Autodesk Inventor part; units mm, degrees
ref_plane "YZ Plane" through (0, 0, 0) normal (1, 0, 0) x (0, 1, 0)
ref_plane "XZ Plane" through (0, 0, 0) normal (0, 1, 0) x (-1, 0, 0)
ref_plane "XY Plane" through (0, 0, 0) normal (0, 0, 1) x (1, 0, 0)
sketch "Sketch1" plane through (0, 0, 0) normal (0, 0, 1) x (1, 0, 0)
  line L0 (-27.3, -5) -> (21, -5)
  line L1 (21, 0) -> (-27.3, 0)
  line L2 (-27.3, 0) -> (-27.3, -5)
  line L3 (17.4, 46.3236) -> (17.4, 0)
  line L4 (17.4, 0) -> (21, 0)
  line L5 (21, 41.8826) -> (21, 41.2832)
  line L6 (17.4, 46.3236) -> (21, 46.3236)
  line L7 (21, 46.3236) -> (21, 0)
  line L8 (21, 0) -> (17.4, 0)
  line L9 (17.4, 0) -> (17.4, 46.3236)
  line L10 (21, 0) -> (21, -5)
  point P0 (0, 0)
  point P1 (-27.3, 0)
  point P2 (17.4, 38.1655)
extrude "Extrusion1" add sketch "Sketch1" against normal blind 15
sketch "Sketch2" plane through (0, 0, 0) normal (0, 0, 1) x (1, 0, 0)
  line L0 (17.4, 0) -> (-27.3, 0)
  line L1 (-27.3, 0) -> (-27.3, -5)
  line L2 (21, -5) -> (21, 46.3236)
  line L3 (21, 46.3236) -> (17.4, 46.3236)
  line L4 (17.4, 46.3236) -> (17.4, 0)
  line L5 (-27.3, -5) -> (21, -5)
  point P0 (0, 0)
extrude "Extrusion2" add sketch "Sketch2" along normal blind 2
sketch "Sketch3" plane through (17.4, 0, -15) normal (-1, 0, 0) x (0, 0, 1)
  line L0 (10.8285, 34.887) -> (11.0682, 35.4658)
  line L1 (11.15, 36.087) -> (11.0682, 35.4658)
  line L2 (11.0682, 36.7082) -> (11.15, 36.087)
  line L3 (10.8285, 37.287) -> (11.0682, 36.7082)
  line L4 (10.4471, 37.7841) -> (10.8285, 37.287)
  line L5 (9.95, 38.1655) -> (10.4471, 37.7841)
  line L6 (9.3712, 38.4052) -> (9.95, 38.1655)
  line L7 (9.3712, 38.4052) -> (8.75, 38.487)
  line L8 (8.1288, 38.4052) -> (8.75, 38.487)
  line L9 (8.1288, 38.4052) -> (7.55, 38.1655)
  line L10 (7.55, 38.1655) -> (7.0529, 37.7841)
  line L11 (7.0529, 37.7841) -> (6.6715, 37.287)
  line L12 (6.6715, 37.287) -> (6.4318, 36.7082)
  line L13 (6.4318, 36.7082) -> (6.35, 36.087)
  line L14 (6.35, 36.087) -> (6.4318, 35.4658)
  line L15 (6.4318, 35.4658) -> (6.6715, 34.887)
  line L16 (6.6715, 34.887) -> (7.0529, 34.3899)
  line L17 (7.0529, 34.3899) -> (7.55, 34.0085)
  line L18 (8.1288, 33.7688) -> (7.55, 34.0085)
  line L19 (8.1288, 33.7688) -> (8.75, 33.687)
  line L20 (8.75, 33.687) -> (9.3712, 33.7688)
  line L21 (9.3712, 33.7688) -> (9.95, 34.0085)
  line L22 (9.95, 34.0085) -> (10.4471, 34.3899)
  line L23 (10.8285, 34.887) -> (10.4471, 34.3899)
  line L24 (8.75, 35.087) -> (9.0088, 35.1211)
  line L25 (8.4912, 35.1211) -> (8.75, 35.087)
  line L26 (8.25, 35.221) -> (8.4912, 35.1211)
  line L27 (8.0429, 35.3799) -> (8.25, 35.221)
  line L28 (7.884, 35.587) -> (8.0429, 35.3799)
  line L29 (7.7841, 35.8282) -> (7.884, 35.587)
  line L30 (7.75, 36.087) -> (7.7841, 35.8282)
  line L31 (7.7841, 36.3458) -> (7.75, 36.087)
  line L32 (7.884, 36.587) -> (7.7841, 36.3458)
  line L33 (8.0429, 36.7941) -> (7.884, 36.587)
  line L34 (8.25, 36.953) -> (8.0429, 36.7941)
  line L35 (8.4912, 37.0529) -> (8.25, 36.953)
  line L36 (8.75, 37.087) -> (8.4912, 37.0529)
  line L37 (8.75, 37.087) -> (9.0088, 37.0529)
  line L38 (9.0088, 37.0529) -> (9.25, 36.953)
  line L39 (9.25, 36.953) -> (9.4571, 36.7941)
  line L40 (9.4571, 36.7941) -> (9.616, 36.587)
  line L41 (9.616, 36.587) -> (9.7159, 36.3458)
  line L42 (9.7159, 36.3458) -> (9.75, 36.087)
  line L43 (9.75, 36.087) -> (9.7159, 35.8282)
  line L44 (9.7159, 35.8282) -> (9.616, 35.587)
  line L45 (9.616, 35.587) -> (9.4571, 35.3799)
  line L46 (9.4571, 35.3799) -> (9.25, 35.221)
  line L47 (9.25, 35.221) -> (9.0088, 35.1211)
  circle A0 centre (8.75, 36.087) radius 2.5
  arc A1 (12.25, 29.4537) -> (5.25, 29.4537) centre (8.75, 36.087) ccw
  line L48 (8.75, 36.087) -> (8.75, 28.587)
  line L49 (0, 0) -> (17, 0)
  line L50 (0, -5) -> (0, 0)
  line L51 (0, -5) -> (17, -5)
  line L52 (17, 0) -> (17, -5)
  line L53 (8.75, 28.587) -> (8.75, 0)
  line L54 (0, 0) -> (17, 0)
  line L55 (5.25, 14.2935) -> (5.25, 28.587)
  line L56 (12.25, 28.587) -> (12.25, 14.2935)
  line L57 (12.25, 0) -> (5.25, 0)
  line L58 (5.25, 0) -> (12.25, 28.587) construction
  line L59 (5.25, 28.587) -> (12.25, 0) construction
  line L60 (12.25, 28.587) -> (12.25, 29.4537)
  line L61 (5.25, 28.587) -> (5.25, 29.4537)
  line L62 (0, 46.3236) -> (17, 46.3236)
  line L63 (17, 46.3236) -> (0, 46.3236)
  line L64 (0, 46.3236) -> (0, 0)
  line L65 (0, 0) -> (17, 0)
  line L66 (17, 0) -> (17, 46.3236)
  line L67 (5.25, 14.2935) -> (0, 0)
  line L68 (12.25, 14.2935) -> (17, 0)
  point P0 (15, 0)
  point P1 (8.75, 14.2935)
  dimension "d6" = 5
  dimension "d7" = 15
  dimension "d8" = 7
extrude "Extrusion3" cut sketch "Sketch3" against normal up to surface (3.6 mm away) contours L25 L26 L27 L28 L29 L30 L31 L32 L33 L34 L35 L36 L37 L38 L39 L40 L41 L42 L43 L44 L45 L46 L47 L24 | L23 L22 L21 L20 L19 L18 L17 L16 L15 L14 L13 L12 L11 L10 L9 L8 L7 L6 L5 L4 L3 L2 L1 L0 | L64 L62 L66 L68 L56 L60 A1 L61 L55 L67
sketch "Sketch5" plane through (-27.3, -5, -15) normal (0, -1, 0) x (1, 0, 0)
  line L0 (4.8, 15) -> (4.8, 2.5)
  line L1 (27.3, 15) -> (4.8, 15)
  line L2 (27.3, 2.5) -> (27.3, 15)
  line L3 (27.3, 2.5) -> (4.8, 2.5)
  line L4 (4.8, 2.5) -> (27.3, 15)
  line L5 (27.55, 2.25) -> (4.55, 2.25)
  line L6 (4.55, 2.25) -> (4.55, 15.25)
  line L7 (4.55, 15.25) -> (27.55, 15.25)
  line L8 (27.55, 15.25) -> (27.55, 2.25)
  line L9 (27.55, 2.25) -> (4.55, 15.25) construction
  line L10 (4.55, 2.25) -> (27.55, 15.25) construction
  line L11 (27.55, 5.75) -> (31.05, 5.75)
  line L12 (31.05, 5.75) -> (31.05, 11.75)
  line L13 (31.05, 11.75) -> (27.55, 11.75)
  line L14 (24.05, 5.75) -> (31.05, 11.75) construction
  line L15 (31.05, 5.75) -> (24.05, 11.75) construction
  point P0 (16.05, 8.75)
  point P1 (27.55, 8.75)
  dimension "d11" = 23
  dimension "d12" = 13
  dimension "d13" = 7
  dimension "d14" = 6
extrude "Extrusion4" cut sketch "Sketch5" against normal up to surface (5 mm away) contours L1 L4 L0 | L4 L2 L3 | L5 L6 L7 L8 | L8 L13 L12 L11
properties part number "arm"
Part model, mm, in its own coordinate system. A direction names the side the tool comes from. Round coordinates to 2 decimals unless told otherwise and drop trailing zeros. Loops run counter-clockwise (first coordinate to the right, second up) from the corner with the lowest first, then second, coordinate; pieces in that order, holes last. Notation, with made-up numbers: (-26, 53.25) -> (32, 53.25) arc R25 ccw to (32, 75.25) -> close; hole circle Ø9 at (-2, 2). An arc over 180 degrees is marked (long way). Use a Markdown table: item, result.
1) Cut at C-C, the plane y = 27. List the corners of the cut face in (x, z), and give its area (3 significant figures).
The answers:
| item | result |
|---|---|
| outline | (17.4, -9.75) -> (21, -9.75) -> (21, -2.75) -> (17.4, -2.75) -> close |
| area | 25.2 mm2 |
2) Tool access for faces 1 (the flat face through (17.4, 22, -7)), 2 (the flat face through (19, 22, -2.75)), 3 (the flat face through (-22.75, -3, -6)), 4 (the flat face through (19.175, 7.247, -12.338)), 5 (the cylindrical face through (19.17, 43.58, -5.97)): list every direction of +Z, -Z, +X, -X, +Y, -Y with a clear straight run to the whole face (end or side of a thin tool).
The answers:
| item | result |
|---|---|
| face 1 | +Z, -Z, -X, +Y |
| face 2 | +Z, +X, -X |
| face 3 | +Y, -Y |
| face 4 | -Z, +X, -X |
| face 5 | +X, -X |
3) Probe line 1 (Z direction, x = -15.5, y = -1); line 2 (X direction, y = -2, z = -0.5); line 3 (X direction, y = 6, z = -3.75). List the from-to ranges inside material, lowest first. Write a range as [from, to].
The answers:
| item | result |
|---|---|
| line 1 | z = [-15, -12.75], [0.25, 2] |
| line 2 | x = [-27.3, -22.75], [0.25, 21] |
| line 3 | x = [17.4, 21] |
4) Drop flat-ended pins along their axis: pin 1 Ø8 at (x, y) = (12, 28) entering from +Z; pin 2 Ø1 at (x, z) = (6.5, -9) entering from +Y; pin 3 Ø3 at (x, y) = (19, 21) entering from +Z; pin 4 Ø4 at (x, y) = (18.5, 19.5) entering from -Z. Give the stop position or say it passes through.
The answers:
| item | result |
|---|---|
| pin 1 | passes through |
| pin 2 | stops at y = 0 |
| pin 3 | stops at z = -2.75 |
| pin 4 | stops at z = -9.75 |
5) Cut at A-A, the plane x = -0.5. List the corners of the cut face in (y, z).
The answers:
| item | result |
|---|---|
| outline | (-5, -15) -> (0, -15) -> (0, -12.75) -> (-5, -12.75) -> close; (-5, 0.25) -> (0, 0.25) -> (0, 2) -> (-5, 2) -> close |
6) Cut at B-B, the plane x = 8. List the corners of the cut face in (y, z), and give its area (3 significant figures).
The answers:
| item | result |
|---|---|
| outline | (-5, -15) -> (0, -15) -> (0, 2) -> (-5, 2) -> close |
| area | 85.0 mm2 |
7) Pull direction Z, two halves, no side cores. Call faces 6 (the flat face through (-3, -2, 2)), 7 (the flat face through (-3, -2, -15)), 8 (the flat face through (3.75, -3, -6)): pulls with the +Z half, pulls with the -Z half, needs draft (parallel to the pull), parting line crosses it, or undercut.
The answers:
| item | result |
|---|---|
| face 6 | pulls with the +Z half |
| face 7 | pulls with the -Z half |
| face 8 | undercut |
